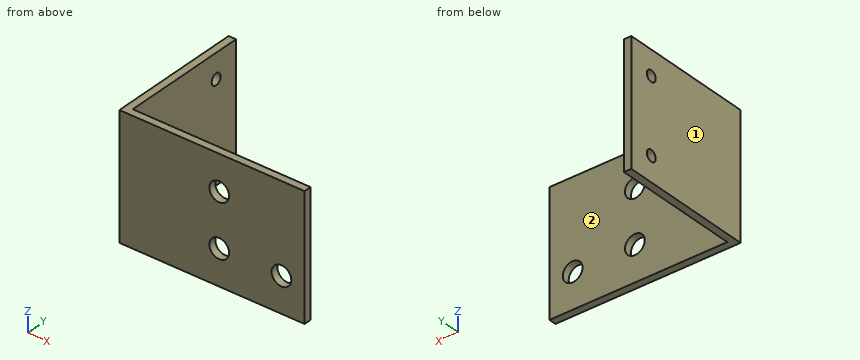
from build123d import *

# Parameters (mm, degrees)
EXTRUDE_1_DEPTH     = 50
SKETCH_6_R          = 2
CUT_EXTRUDE_2_DEPTH = 4
SKETCH1_R           = 2
CUT_EXTRUDE1_DEPTH  = 4
SKETCH2_R           = 4
CUT_EXTRUDE2_DEPTH  = 4
SKETCH4_R           = 2.25
CUT_EXTRUDE3_DEPTH  = 76


with BuildPart() as part:
    # Эскиз1 → Бобышка-Вытянуть1 (new body)
    with BuildSketch(Plane.XY):
        Polygon((0, 0), (75, 0), (75, 3), (3, 3), (3, 55), (0, 55), align=None)
    extrude(amount=EXTRUDE_1_DEPTH)

    # Эскиз6 → Вырез-Вытянуть2 (cut, through all)
    with BuildSketch(Plane(origin=(0, 3, 0), x_dir=(1, 0, 0), z_dir=(0, 1, 0))):
        with Locations((40.4, -14.3)):
            Circle(SKETCH_6_R)
        with Locations((40.4, -35.7)):
            Circle(SKETCH_6_R)
    extrude(amount=-CUT_EXTRUDE_2_DEPTH, mode=Mode.SUBTRACT)

    # Sketch1 → Cut-Extrude1 (cut, through all)
    with BuildSketch(Plane(origin=(0, 3, 0), x_dir=(1, 0, 0), z_dir=(0, 1, 0))):
        with Locations((65.6, -14.3)):
            Circle(SKETCH1_R)
    extrude(amount=-CUT_EXTRUDE1_DEPTH, mode=Mode.SUBTRACT)

    # Sketch2 → Cut-Extrude2 (cut, through all)
    with BuildSketch(Plane(origin=(0, 3, 0), x_dir=(1, 0, 0), z_dir=(0, 1, 0))):
        with Locations((40.4, -14.3)):
            Circle(SKETCH2_R)
        with Locations((65.6, -14.3)):
            Circle(SKETCH2_R)
        with Locations((40.4, -35.7)):
            Circle(SKETCH2_R)
    extrude(amount=-CUT_EXTRUDE2_DEPTH, mode=Mode.SUBTRACT)

    # Sketch4 → Cut-Extrude3 (cut, through all)
    with BuildSketch(Plane.ZY):
        with Locations((10, 45)):
            Circle(SKETCH4_R)
        with Locations((40, 45)):
            Circle(SKETCH4_R)
    extrude(amount=-CUT_EXTRUDE3_DEPTH, mode=Mode.SUBTRACT)


solid = part.part
Source: CAD feature listing. Evaluate the final solid. Frame: model axes, mm. Face numbers are marked on the shaded views. A direction names the side the tool comes from. Give positions to 0.01 mm unless a question says otherwise; leave off trailing zeros. Write each loop counter-clockwise with the first axis right and the second up, starting at its lowest first coordinate (ties: lowest second). Pieces come first, ordered by that corner, then holes. Notation, with made-up numbers: (52, 44.25) - (81, 44.25) arc R17 cw to (81, 58.25) - close; hole circle Ø6 at (84.5, 61). An arc over 180 degrees is marked (long way). Write item = value, one per line. Start each with the question number.
Q1. Reachability of the marked faces 1 and 2 from +Z, -Z, +X, -X, +Y, -Y: full face, straight path, thin tool, end or side. Return the list, or none.
Q2. Cut plane D-D, the plane z = 14.3. Return loops of the section in (x, y).
Q3. Cut plane A-A, the plane z = 35.7. Return loops of the section in (x, y), then the cut area to 3 significant figures.
Q4. Material intervals for probe 1 along Z at (x, y) = (40.4, 2.1); probe 2 along Y at (x, z) = (1.55, 10); probe 3 along X at (y, z) = (1, 14), sorted ascending.
Q5. Cut plane C-C, the plane x = 40.4. Return loops of the section in (y, z).
Q6. Pin query (flat end, axial travel): pin 1 Ø12 at (x, z) = (16.5, 13.5) entering from +Y; pin 2 Ø5 at (y, z) = (43.5, 22.5) entering from +X. Return the tip coordinate at first contact, or that it passes through.
Q7. Cut plane B-B, the plane x = 65.6. Return loops of the section in (y, z).
Computed values:
q1.face_1 = +Z, -Z, -X, +Y, -Y
q1.face_2 = +Z, -Z, +X, +Y
q2.outline = (0, 0) - (36.4, 0) - (36.4, 3) - (3, 3) - (3, 55) - (0, 55) - close; (44.4, 0) - (61.6, 0) - (61.6, 3) - (44.4, 3) - close; (69.6, 0) - (75, 0) - (75, 3) - (69.6, 3) - close
q3.outline = (0, 0) - (36.4, 0) - (36.4, 3) - (3, 3) - (3, 55) - (0, 55) - close; (44.4, 0) - (75, 0) - (75, 3) - (44.4, 3) - close
q3.area = 357 mm²
q4.probe_1 = 0 to 10.3, 18.3 to 31.7, 39.7 to 50
q4.probe_2 = 0 to 42.75, 47.25 to 55
q4.probe_3 = 0 to 36.41, 44.39 to 61.61, 69.59 to 75
q5.outline = (0, 0) - (3, 0) - (3, 10.3) - (0, 10.3) - close; (0, 18.3) - (3, 18.3) - (3, 31.7) - (0, 31.7) - close; (0, 39.7) - (3, 39.7) - (3, 50) - (0, 50) - close
q6.pin_1 = 3
q6.pin_2 = 3
q7.outline = (0, 0) - (3, 0) - (3, 10.3) - (0, 10.3) - close; (0, 18.3) - (3, 18.3) - (3, 50) - (0, 50) - close
